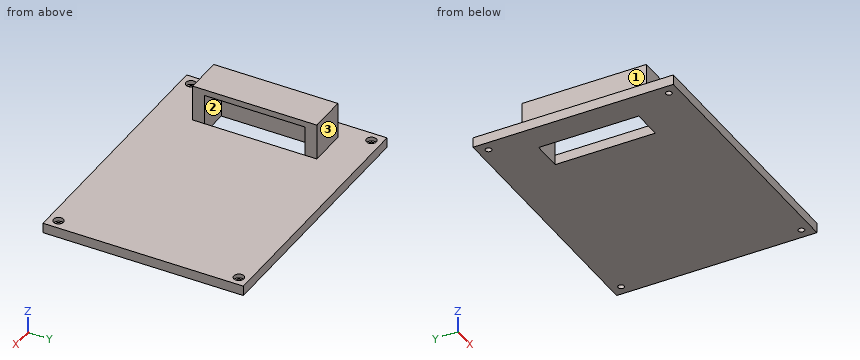
from build123d import *

# Parameters (mm, degrees)
SKETCH082_W     = 130
SKETCH082_H     = 100
PAD013_DEPTH    = 5
SKETCH083_W     = 19
SKETCH083_H     = 62
PAD014_DEPTH    = 18
SKETCH084_W     = 15
SKETCH084_H     = 50
POCKET068_DEPTH = 20
SKETCH085_R     = 1.5
POCKET069_DEPTH = 5
SKETCH086_R     = 2.5
POCKET070_DEPTH = 2


with BuildPart() as part:
    # Sketch082 → Pad013 (new body)
    with BuildSketch(Plane.XY):
        with Locations((65, 50)):
            Rectangle(SKETCH082_W, SKETCH082_H)
    extrude(amount=PAD013_DEPTH)

    # Sketch083 (on Face6 of Pad013) → Pad014 (join)
    with BuildSketch(Plane.XY.offset(5)):
        with Locations((19.5, 50)):
            Rectangle(SKETCH083_W, SKETCH083_H)
    extrude(amount=PAD014_DEPTH)

    # Sketch084 (on Face4 of Pad014) → Pocket068 (cut)
    with BuildSketch(Plane(origin=(0, 0, 0), x_dir=(1, 0, 0), z_dir=(0, 0, -1))):
        with Locations((21.5, -50)):
            Rectangle(SKETCH084_W, SKETCH084_H)
    extrude(amount=-POCKET068_DEPTH, mode=Mode.SUBTRACT)

    # Sketch085 (on Face4 of Pocket068) → Pocket069 (cut)
    with BuildSketch(Plane(origin=(0, 0, 0), x_dir=(1, 0, 0), z_dir=(0, 0, -1))):
        with Locations((5, -5)):
            Circle(SKETCH085_R)
        with Locations((125, -5)):
            Circle(SKETCH085_R)
        with Locations((5, -95)):
            Circle(SKETCH085_R)
        with Locations((125, -95)):
            Circle(SKETCH085_R)
    extrude(amount=-POCKET069_DEPTH, mode=Mode.SUBTRACT)

    # Sketch086 (on Face5 of Pocket069) → Pocket070 (cut)
    with BuildSketch(Plane.XY.offset(5)):
        with Locations((5, 95)):
            Circle(SKETCH086_R)
        with Locations((5, 5)):
            Circle(SKETCH086_R)
        with Locations((125, 5)):
            Circle(SKETCH086_R)
        with Locations((125, 95)):
            Circle(SKETCH086_R)
    extrude(amount=-POCKET070_DEPTH, mode=Mode.SUBTRACT)


with BuildPart() as part_1:
    # Body013 placement: moved
    add(part.part.moved(Location((0, 0, 45))))


solid = part_1.part
Input: part model. Units: mm. Frame: model coordinates. Face numbers are marked on the shaded views. Round coordinates to 2 decimals unless told otherwise and drop trailing zeros. Order: outer loops, then holes, each group sorted by start corner. A loop starts at its lowest first (then second) coordinate and runs counter-clockwise, first axis right, second up.
1. Cut plane D-D, the plane z = 54.5. Output: boundary loops of the cut face in (x, y), then the cut area to 3 significant figures.
The answers:
outline: (10, 19) - (29, 19) - (29, 25) - (14, 25) - (14, 75) - (29, 75) - (29, 81) - (10, 81) - close
area: 428 mm2
2. Cut plane C-C, the plane y = 40.5. Output: boundary loops of the cut face in (x, z), then the cut area to 3 significant figures.
The answers:
outline: (0, 45) - (14, 45) - (14, 65) - (29, 65) - (29, 68) - (10, 68) - (10, 50) - (0, 50) - close; (29, 45) - (130, 45) - (130, 50) - (29, 50) - close
area: 692 mm2
3. Cut plane B-B, the plane x = 5. Output: boundary loops of the cut face in (y, z).
The answers:
outline: (0, 45) - (3.5, 45) - (3.5, 48) - (2.5, 48) - (2.5, 50) - (0, 50) - close; (6.5, 45) - (93.5, 45) - (93.5, 48) - (92.5, 48) - (92.5, 50) - (7.5, 50) - (7.5, 48) - (6.5, 48) - close; (96.5, 45) - (100, 45) - (100, 50) - (97.5, 50) - (97.5, 48) - (96.5, 48) - close
4. Cut plane A-A, the plane y = 5. Output: boundary loops of the cut face in (x, z), then the cut area to 3 significant figures.
The answers:
outline: (0, 45) - (3.5, 45) - (3.5, 48) - (2.5, 48) - (2.5, 50) - (0, 50) - close; (6.5, 45) - (123.5, 45) - (123.5, 48) - (122.5, 48) - (122.5, 50) - (7.5, 50) - (7.5, 48) - (6.5, 48) - close; (126.5, 45) - (130, 45) - (130, 50) - (127.5, 50) - (127.5, 48) - (126.5, 48) - close
area: 612 mm2
5. Pin query (flat end, axial travel): P1, Ø6, axis at x = 62, y = 16, coming from the +Z side; P2, Ø1.5, axis at x = 126, y = 94, coming from the +Z side; P3, Ø2.5, axis at x = 125, y = 5, coming from the +Z side; P4, Ø4.5, axis at x = 125, y = 95, coming from the -Z side. Return the tip coordinate at first contact, or that it passes through.
The answers:
P1: stops at z = 50
P2: stops at z = 48
P3: passes through
P4: stops at z = 45
6. Material intervals for line 1 (Y direction, x = 5, z = 46.55); line 2 (Y direction, x = 125, z = 49.6); line 3 (Y direction, x = 27, z = 46), sorted ascending.
The answers:
line 1: y = 0 to 3.5, 6.5 to 93.5, 96.5 to 100
line 2: y = 0 to 2.5, 7.5 to 92.5, 97.5 to 100
line 3: y = 0 to 25, 75 to 100
7. Mould query, pull axis Y, two halves, no side actions, for the marked faces 1, 2 and 3. Classes: released by +Y, released by -Y, zero draft, split by the parting line, or undercut.
The answers:
face 1: zero draft
face 2: undercut
face 3: released by +Y
